Work out the finished part from the listing and answer in its coordinate system (mm). Face numbers are marked on the shaded views. A direction names the side the tool comes from. Round coordinates to 2 decimals unless told otherwise and drop trailing zeros. Loops run counter-clockwise (first coordinate to the right, second up) from the corner with the lowest first, then second, coordinate; pieces in that order, holes last. Notation, with made-up numbers: (-37.75, -23) - (-2.75, -23) arc R18 ccw to (-2.75, -18) - close; hole circle Ø7 at (83.5, 35.5). An arc over 180 degrees is marked (long way). Answer as CSV lines item,"result". Start each with the question number.
Q1. Section B-B on x = 10 is taken. Write down the section's boundary in (y, z).
Q2. Section D-D on z = -16 is taken. Write down the section's boundary in (x, y), then the cut area to 3 significant figures.
Q3. Section C-C on y = 78 is taken. Write down the section's boundary in (x, z), then the cut area to 3 significant figures.
Q4. For the marked faces 4, 5 and 6, determine the directions among +Z, -Z, +X, -X, +Y, -Y from which every point of the face is accessible in a straight line to the end or side of a thin tool.
Q5. Section A-A on z = -10 is taken. Write down the section's boundary in (x, y), then the cut area to 3 significant figures.
Q6. The mould has two halves that part along Z. Classify the marked faces 1, 2 and 3: +Z half, -Z half, draft (parallel to the pull), parting line (faces both ways), or undercut.
Q7. Straight lines are drawn through the part: L1, parallel to Z at x = 25, y = 20.5; L2, parallel to X at y = 0.6, z = -10; L3, parallel to Y at x = 39.4, z = -10. For each, find the intervals that lie inside material, in ascending order. Write a range as [from, to].
Q8. Each of these flat-tipped pins is pushed along its axis until it touches: pin 1 Ø1 at (x, z) = (36, -4) entering from -Y; pin 2 Ø5.5 at (x, z) = (10, -10) entering from -Y; pin 3 Ø1 at (y, z) = (77, -17) entering from -X; pin 4 Ø6 at (x, z) = (29.5, -14.5) entering from +Y. Where does it stop, or does it pass through?
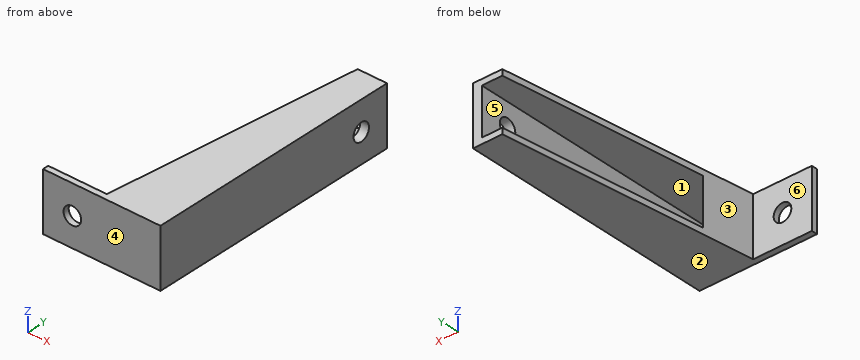
```python
from build123d import *

# Parameters (mm, degrees)
SKETCH1_W           = 40
SKETCH1_H           = 20
BOSS_EXTRUDE1_DEPTH = 2
SKETCH2_R           = 3
CUT_EXTRUDE1_DEPTH  = 2
SKETCH3_W           = 20
SKETCH3_H           = 20
SKETCH3_W_2         = 15
SKETCH3_H_2         = 16
BOSS_EXTRUDE2_DEPTH = 86
SKETCH4_R           = 3
CUT_EXTRUDE2_DEPTH  = 86
CUT_EXTRUDE3_DEPTH  = 86


with BuildPart() as part:
    # Sketch1 → Boss-Extrude1 (new body)
    with BuildSketch(Plane(origin=(0, 0, 0), x_dir=(1, 0, 0), z_dir=(0, 1, 0))):
        with Locations((20, 10)):
            Rectangle(SKETCH1_W, SKETCH1_H)
    extrude(amount=BOSS_EXTRUDE1_DEPTH)

    # Sketch2 → Cut-Extrude1 (cut)
    with BuildSketch(Plane(origin=(0, 2, 0), x_dir=(1, 0, 0), z_dir=(0, 1, 0))):
        with Locations(Location((10, 10, 0), (0, 0, 270))):
            Circle(SKETCH2_R)
    extrude(amount=-CUT_EXTRUDE1_DEPTH, mode=Mode.SUBTRACT)

    # Sketch3 → Boss-Extrude2 (add)
    with BuildSketch(Plane(origin=(0, 2, 0), x_dir=(1, 0, 0), z_dir=(0, 1, 0))):
        with Locations((30, 10)):
            Rectangle(SKETCH3_W, SKETCH3_H)
        with Locations((29.5, 10)):
            Rectangle(SKETCH3_W_2, SKETCH3_H_2, mode=Mode.SUBTRACT)
    extrude(amount=BOSS_EXTRUDE2_DEPTH)

    # Sketch4 → Cut-Extrude2 (cut)
    with BuildSketch(Plane(origin=(40, 0, 0), x_dir=(0, 0, -1), z_dir=(1, 0, 0))):
        with Locations((10, 78)):
            Circle(SKETCH4_R)
    extrude(amount=-CUT_EXTRUDE2_DEPTH, mode=Mode.SUBTRACT)

    # Sketch5 → Cut-Extrude3 (cut)
    with BuildSketch(Plane.XY):
        Polygon((30, 88), (20, 2), (20, 88), align=None)
    extrude(amount=-CUT_EXTRUDE3_DEPTH, mode=Mode.SUBTRACT)


solid = part.part
```
Findings:
1,outline,"(0, -20) - (2, -20) - (2, -13) - (0, -13) - close; (0, -7) - (2, -7) - (2, 0) - (0, 0) - close"
2,outline,"(0, 0) - (40, 0) - (40, 88) - (37, 88) - (37, 2) - (22, 2) - (22, 19.2) - (20, 2) - (0, 2) - close"
2,area,"355 mm^2"
3,outline,"(28.84, -20) - (40, -20) - (40, -13) - (37, -13) - (37, -18) - (28.84, -18) - close; (28.84, -2) - (37, -2) - (37, -7) - (40, -7) - (40, 0) - (28.84, 0) - close"
3,area,"74.7 mm^2"
4,face 4,"+Z, -Z, +X, -X, -Y"
4,face 5,"+Y"
4,face 6,"+Z, -Z, -X, +Y"
5,outline,"(0, 0) - (7, 0) - (7, 2) - (0, 2) - close; (13, 0) - (40, 0) - (40, 75) - (37, 75) - (37, 2) - (22, 2) - (22, 19.2) - (20, 2) - (13, 2) - close; (37, 81) - (40, 81) - (40, 88) - (37, 88) - close"
5,area,"325 mm^2"
6,face 1,"undercut"
6,face 2,"-Z half"
6,face 3,"draft"
7,L1,"z = [-20, -18], [-2, 0]"
7,L2,"x = [0, 7], [13, 40]"
7,L3,"y = [0, 75], [81, 88]"
8,pin 1,"stops at y = 0"
8,pin 2,"passes through"
8,pin 3,"stops at x = 37"
8,pin 4,"stops at y = 2"
